Check sheet for the modelled part. Datum: model origin and axes. Units: mm. A direction names the side the tool comes from. Give positions to 0.01 mm unless a question says otherwise; leave off trailing zeros. Write each loop counter-clockwise with the first axis right and the second up, starting at its lowest first coordinate (ties: lowest second). Pieces come first, ordered by that corner, then holes. Notation, with made-up numbers: M 37.25,68 L 68.25,68 A28 ccw 68.25,94 Z; hole C 27.25,89.25 d8. An arc over 180 degrees is marked long. One line per item, written item: value. Start each with the question number.
from build123d import *

# Parameters (mm, degrees)
F0_W     = 40
F0_H     = 310
F1_DEPTH = 820
F2_T     = -3
F3_R     = 2.5
F4_DEPTH = 820.001


with BuildPart() as f1:
    # F0 (on Top) → F1 (new body)
    with BuildSketch(Plane.XY):
        with Locations((-20, 59.262322)):
            Rectangle(F0_W, F0_H)
    extrude(amount=F1_DEPTH)

    # F2
    f2_openings = [f1.faces().sort_by_distance(p)[0] for p in [
        (-20, 214.262322, 410),
        (-20, -95.737678, 410),
        (-40, 59.262322, 410),
    ]]
    offset(amount=F2_T, openings=f2_openings)

    # F3 (on face) → F4 (cut, through all)
    with BuildSketch(Plane.XY.offset(820)):
        with Locations((-30, 184.262322)):
            Circle(F3_R)
        with Locations((-10, 184.262322)):
            Circle(F3_R)
        with Locations((-30, -65.737678)):
            Circle(F3_R)
        with Locations((-10, -65.737678)):
            Circle(F3_R)
    extrude(amount=-F4_DEPTH, mode=Mode.SUBTRACT)


solid = f1.part
1) Cross-section at B-B (z = 619.5). Record the boundary of the cut face in (x, y), plus the area to 3 significant figures.
2) Gauge pin test, flat end, axial feed: pin 1 (3 mm diameter, centred on y = 78, z = 171.5, fed in from -X). Record the tip position at first contact, or that the pin passes through.
3) Tool access check on faces 4 (the flat face through (-3, 57, 404)), 5 (the flat face through (-20, 61, 820)). Record the directions out of +Z, -Z, +X, -X, +Y, -Y that give a thin tool (end or side, any length) a straight path to the whole face; none if there is none.
4) Cross-section at A-A (y = 165). Record the boundary of the cut face in (x, z), plus the area to 3 significant figures.
5) Material ranges on L1, parallel to Y at x = -10, z = 818; L2, parallel to Z at x = -14, y = -73.5; L3, parallel to X at y = -51, z = 134, recorded low to high. Write a range as from..to.
6) Draft check along Z on faces 1 (the flat face through (-20, 61, 0)), 2 (the flat face through (-1, -95.738, 408)), 3 (the flat face through (-22, 61, 817)). Enter one of: released by +Z, released by -Z, zero draft, split by the parting line, or undercut.
Data:
1. outline: M -3,-95.74 L 0,-95.74 L 0,214.26 L -3,214.26 Z
1. area: 930 mm2
2. pin 1: stops at x = -3
3. face 4: -X, +Y, -Y
3. face 5: +Z, +X, -X, +Y, -Y
4. outline: M -40,0 L 0,0 L 0,820 L -40,820 L -40,817 L -3,817 L -3,3 L -40,3 Z
4. area: 2,680 mm2
5. L1: y = -95.74..-68.24, -63.24..181.76, 186.76..214.26
5. L2: z = 0..3, 817..820
5. L3: x = -3..0
6. face 1: released by -Z
6. face 2: zero draft
6. face 3: undercut
